Could you check a few things on this drawing? It's one solid part, dimensions in mm from its lowest x, y, z. Coordinates: 2 decimals unless noted, no trailing zeros. Loops run counter-clockwise (first coordinate to the right, second up) from the corner with the lowest first, then second, coordinate; pieces in that order, holes last. Notation, with made-up numbers: M 73.5,4.5 L 108.5,4.5 A37 cw 108.5,43.5 Z; hole C 47.25,-8.5 d10. An arc over 180 degrees is marked long. Answer as a JSON object with one key per item and string values. Group by question number.
Item 1: I'm going to push flat-ended pins straight in: pin 1 Ø1 at (x, z) = (62.5, 4.5) entering from -Y; pin 2 Ø3 at (x, z) = (3, 5) entering from -Y; pin 3 Ø5 at (y, z) = (14, 5.5) entering from +X; pin 4 Ø1 at (y, z) = (65.5, 7.5) entering from -X. Where does each tip first touch, or does it pass through?
Item 2: If I drill on line 1 (X direction, y = 71.5, z = 4.75); line 2 (Y direction, x = 24.5, z = 2.5); line 3 (Y direction, x = 73.5, z = 3.5), over which ranges is the centre line in solid material (lowest first)?
Item 3: Suppose I cut it at C-C (x = 103.5). Write out the boundary of the cut face in (y, z).
Item 4: Suppose I cut it at B-B (y = 57.5). Write out the boundary of the cut face in (x, z), then the cut area to 3 significant figures.
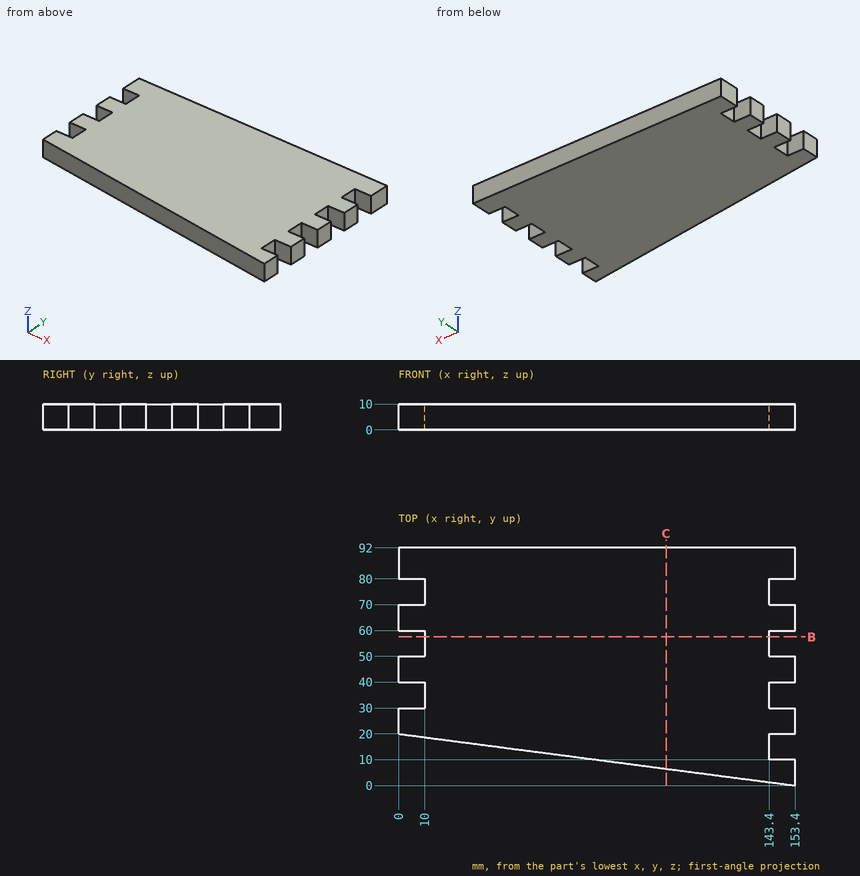
From the geometry:
{
 "1": {"pin 1": "y = 11.79", "pin 2": "y = 19.41", "pin 3": "x = 143.4", "pin 4": "x = 0"},
 "2": {"line 1": "10 to 143.4", "line 2": "16.81 to 92", "line 3": "10.42 to 92"},
 "3": {"outline": "M 6.51,0 L 92,0 L 92,10 L 6.51,10 Z"},
 "4": {"outline": "M 10,0 L 143.4,0 L 143.4,10 L 10,10 Z", "area": "1,330 mm2"}
}
